Autodesk Inventor part; units mm, degrees
ref_plane "YZ Plane" through (0, 0, 0) normal (1, 0, 0) x (0, 1, 0)
ref_plane "XZ Plane" through (0, 0, 0) normal (0, 1, 0) x (-1, 0, 0)
ref_plane "XY Plane" through (0, 0, 0) normal (0, 0, 1) x (1, 0, 0)
sketch "Sketch1" plane through (0, 0, 0) normal (0, 0, 1) x (1, 0, 0)
  line L0 (0, 0) -> (0, 6)
  line L1 (0, 6) -> (1.5, 6)
  line L2 (1.5, 6) -> (1.5, 5)
  line L3 (1.5, 5) -> (6.5, 5)
  line L4 (6.5, 5) -> (6.5, 0)
  line L5 (6.5, 0) -> (0, 0)
  dimension "d0" = 10
  dimension "d1" = 12
  dimension "d2" = 1.5
  dimension "d17" = 5
revolve "Revolution1" add sketch "Sketch1" angle 360 about axis through (6.5, 0, 0) along (-1, 0, 0)
sketch "Sketch2" plane through (0, 0, 0) normal (-1, 0, 0) x (0, 0, 1)
  circle A0 centre (0, 0) radius 6
  circle A1 centre (-3.5, 0) radius 0.6
  circle A2 centre (3.5, 0) radius 0.6
  line L0 (-3.5, 0) -> (3.5, 0) construction
  circle A3 centre (0, 0) radius 3.5 construction
  circle A4 centre (0, 0) radius 5 construction
  point P0 (0, 0)
  dimension "d6" = 7
  dimension "d5" = 1.2
  dimension "d7" = 10
extrude "Extrusion1" cut sketch "Sketch2" against normal through all contours A1 | A2
hole "Hole1" at (0, 0, 0) direction (1, 0, 0) diameter 3.2 depth 25
sketch "Sketch3" plane through (0, 0, 0) normal (0, 0, 1) x (1, 0, 0)
  circle A0 centre (2.3333, -3.5) radius 0.5
  line L0 (1.5, -5) -> (6.5, -5) construction
  line L1 (1.5, 5) -> (6.5, 5) construction
  line L2 (-1.3, 0) -> (7.8, 0) construction
  line L3 (1.5, -5) -> (6.5, -5) construction
  line L4 (4, -5) -> (4, 5) construction
  line L5 (1.5, 5) -> (6.5, 5) construction
  point P0 (0, 0)
  dimension "d18" = 1
  dimension "d19" = 3.5
  dimension "d22" = 2.5
  dimension "d23" = 1.6667
extrude "Extrusion2" cut sketch "Sketch3" along normal through all both and the other way through all
equation "\"d23\" = 0.666667 * d22"
properties part number "Capston_Tensioning"
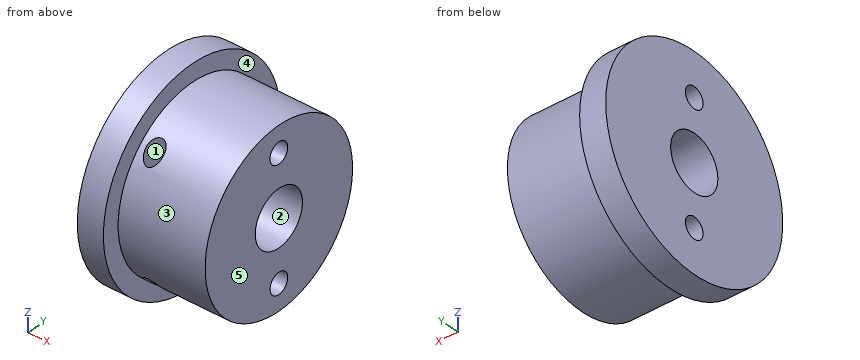
Geometry: final body of the model. Coordinates: model frame, mm. Face numbers are marked on the shaded views. A direction names the side the tool comes from. Give positions to 0.01 mm unless a question says otherwise; leave off trailing zeros. Write each loop counter-clockwise with the first axis right and the second up, starting at its lowest first coordinate (ties: lowest second). Pieces come first, ordered by that corner, then holes.
(1) Ray query, line 1 (Z direction, x = 5, y = 0.25); line 2 (Y direction, x = 2, z = 0); line 3 (X direction, y = -3.5, z = 0.5). Return the intervals inside material, ascending.
(2) First-contact query: P1, Ø6, axis at y = -0.5, z = -2.5, coming from the -X side; P2, Ø1.5, axis at x = 1.5, z = -4.5, coming from the -Y side; P3, Ø1.5, axis at x = 2, z = -2.5, coming from the +Y side; P4, Ø3, axis at x = 3.5, z = -1.5, coming from the -Y side. Flat tips, straight axial feed; report the tip coordinate or a pass-through.
(3) Cut plane C-C, the plane y = -3.5. Return loops of the section in (x, z).
(4) Cut plane B-B, the plane y = 0. Return loops of the section in (x, z).
(5) Cut plane D-D, the plane x = 5.5. Return loops of the section in (y, z).
(6) Cut plane A-A, the plane z = 0. Return loops of the section in (x, y), then the cut area to 3 significant figures.
(7) Access query for the marked faces 4 and 5. Directions: +Z, -Z, +X, -X, +Y, -Y. A direction counts if a zero-diameter tool reaches every point of the face in a straight line with its end or side. Return the directions, or none.
(8) Mould query, pull axis Z, two halves, no side actions, for the marked faces 1, 2 and 3. Classes: released by +Z, released by -Z, zero draft, split by the parting line, or undercut.
Values follow:
1. line 1: z = -4.99 to -4.05, -2.95 to -1.58, 1.58 to 2.95, 4.05 to 4.99
1. line 2: y = -5 to -3.87, -3.13 to -1.6, 1.6 to 5
1. line 3: x = 0 to 1.83, 2.83 to 6.5
2. P1: stops at x = 0
2. P2: stops at y = -4.68
2. P3: stops at y = 5.68
2. P4: stops at y = -5
3. outline: (0, -4.87) - (1.5, -4.87) - (1.5, -3.57) - (1.83, -3.57) - (1.83, 3.57) - (1.5, 3.57) - (1.5, 4.87) - (0, 4.87) - close; (2.83, -3.57) - (6.5, -3.57) - (6.5, 3.57) - (2.83, 3.57) - close
4. outline: (0, -6) - (1.5, -6) - (1.5, -5) - (6.5, -5) - (6.5, -4.1) - (0, -4.1) - close; (0, -2.9) - (6.5, -2.9) - (6.5, -1.6) - (0, -1.6) - close; (0, 1.6) - (6.5, 1.6) - (6.5, 2.9) - (0, 2.9) - close; (0, 4.1) - (6.5, 4.1) - (6.5, 5) - (1.5, 5) - (1.5, 6) - (0, 6) - close
5. outline: circle Ø10 at (0, 0); hole circle Ø3.2 at (0, 0); hole circle Ø1.2 at (0, -3.5); hole circle Ø1.2 at (0, 3.5)
6. outline: (0, -6) - (1.5, -6) - (1.5, -5) - (6.5, -5) - (6.5, -1.6) - (0, -1.6) - close; (0, 1.6) - (6.5, 1.6) - (6.5, 5) - (1.5, 5) - (1.5, 6) - (0, 6) - close; hole circle Ø1 at (2.33, -3.5)
6. area: 46.4 mm2
7. face 4: +X
7. face 5: +Z, -Z, +X, +Y, -Y
8. face 1: zero draft
8. face 2: undercut
8. face 3: split by the parting line
